Autodesk Inventor part; units mm, degrees
ref_plane "YZ Plane" through (0, 0, 0) normal (1, 0, 0) x (0, 1, 0)
ref_plane "XZ Plane" through (0, 0, 0) normal (0, 1, 0) x (-1, 0, 0)
ref_plane "XY Plane" through (0, 0, 0) normal (0, 0, 1) x (1, 0, 0)
sketch "Sketch1" plane through (0, 0, 0) normal (0, 1, 0) x (-1, 0, 0)
  line L0 (0, 0) -> (58.9854, 49.4946)
  line L1 (0, 0) -> (77, 0) construction
  line L2 (58.9854, 49.4946) -> (54.9037, 54.359)
  line L3 (54.9037, 54.359) -> (0, 8.2893)
  line L4 (0, 8.2893) -> (0, 0)
  dimension "d0" = 77
  dimension "d1" = 40
  dimension "d2" = 6.35
extrude "Extrusion1" add sketch "Sketch1" along normal blind 6.35
sketch "Sketch2" plane through (0, 6.35, 0) normal (0, 1, 0) x (1, 0, 0)
  line L0 (-58.9854, -49.4946) -> (-54.9037, -54.359)
  line L1 (-54.9037, -54.359) -> (-58.9854, -49.4946)
  line L2 (-58.9854, -49.4946) -> (-53.6231, -44.9951)
  line L3 (0, 0) -> (-58.9854, -49.4946)
  line L4 (-54.9037, -54.359) -> (0, -8.2893)
  line L5 (-49.5414, -49.8595) -> (-54.9037, -54.359)
  line L6 (-49.5414, -49.8595) -> (-46.4772, -47.2884)
  line L7 (-46.4772, -47.2884) -> (-50.5589, -42.424)
  line L8 (-50.5589, -42.424) -> (-58.9854, -49.4946)
  dimension "d5" = 7
  dimension "d6" = 4
extrude "Extrusion2" cut sketch "Sketch2" against normal blind 10
sketch "Sketch3" plane through (0, 6.35, 0) normal (0, 1, 0) x (1, 0, 0)
  line L0 (0, 0) -> (-50.5589, -42.424)
  line L1 (-50.5589, -42.424) -> (-51.325, -43.0668)
  line L2 (-51.325, -43.0668) -> (-47.2433, -47.9312)
  line L3 (-46.4772, -47.2884) -> (0, -8.2893)
  line L4 (-47.2433, -47.9312) -> (-46.4772, -47.2884)
  line L5 (-46.4772, -47.2884) -> (-50.5589, -42.424)
  dimension "d9" = 1
  dimension "d10" = 6.35
extrude "Extrusion3" add sketch "Sketch3" against normal blind 6.35
properties part number "2ndFloorOAngle"
Source: CAD feature listing. Evaluate the final solid. Frame: model axes, mm. Coordinates: 2 decimals unless noted, no trailing zeros. Write each loop counter-clockwise with the first axis right and the second up, starting at its lowest first coordinate (ties: lowest second). Pieces come first, ordered by that corner, then holes. Notation, with made-up numbers: M 56.25,-22 L 101.25,-22 A12 ccw 101.25,-10 Z; hole C 63.25,16 d6. An arc over 180 degrees is marked long. Use a Markdown table: item, result.
1) Ray query, L1, parallel to Z at x = -26, y = 4.5; L2, parallel to Z at x = -13, y = 3; L3, parallel to X at y = 1, z = 12. Return the intervals inside material, ascending.
Conclusion:
| item | result |
|---|---|
| L1 | z = 21.82 to 30.11 |
| L2 | z = 10.91 to 19.2 |
| L3 | x = -14.3 to -4.42 |
2) Section C-C, the plane x = -16. Output: boundary loops of the cut face in (y, z), then the cut area to 3 significant figures.
Conclusion:
| item | result |
|---|---|
| outline | M 0,13.43 L 6.35,13.43 L 6.35,21.71 L 0,21.71 Z |
| area | 52.6 mm^2 |
3) Section A-A, the plane y = 2.25. Output: boundary loops of the cut face in (x, z) (3 decimals), then the cut area to 3 significant figures.
Conclusion:
| item | result |
|---|---|
| outline | M -51.325,43.067 L -50.559,42.424 L 0,0 L 0,8.289 L -46.477,47.288 L -47.243,47.931 Z |
| area | 409 mm^2 |
4) Section B-B, the plane z = 21. Output: boundary loops of the cut face in (x, y).
Conclusion:
| item | result |
|---|---|
| outline | M -25.03,0 L -15.15,0 L -15.15,6.35 L -25.03,6.35 Z |
5) First-contact query: pin 1 Ø1 at (x, y) = (-34, 3) entering from +Z; pin 2 Ø2 at (y, z) = (4.5, 41.5) entering from +X. Flat tips, straight axial feed; report the tip coordinate or a pass-through.
Conclusion:
| item | result |
|---|---|
| pin 1 | stops at z = 37.24 |
| pin 2 | stops at x = -38.39 |
